```python
from build123d import *

# Parameters (mm, degrees)
BOSS_EXTRUDE3_DEPTH = 30
BOSS_EXTRUDE5_DEPTH = 13
SKETCH6_R           = 6.5
CUT_EXTRUDE1_DEPTH  = 13
SKETCH7_R           = 7.5
CUT_EXTRUDE2_DEPTH  = 13


with BuildPart() as part:
    # Sketch2 → Boss-Extrude3 (new body)
    with BuildSketch(Plane(origin=(0, 0, 0), x_dir=(0, 0, -1), z_dir=(1, 0, 0))):
        Polygon((0, 0), (0, 37), (-13, 37), (-13, 13), (-43, 13), (-43, 0), align=None)
    extrude(amount=BOSS_EXTRUDE3_DEPTH)

    # Sketch4 → Boss-Extrude5 (add)
    with BuildSketch(Plane(origin=(0, 13, 0), x_dir=(1, 0, 0), z_dir=(0, 1, 0))):
        with BuildLine():
            Line((0, -13), (0, -43))
            Line((0, -43), (-5, -43))
            ThreePointArc((-5, -43), (-20, -28), (-5, -13))
            Line((-5, -13), (0, -13))
        make_face()
    extrude(amount=-BOSS_EXTRUDE5_DEPTH)

    # Sketch6 → Cut-Extrude1 (cut)
    with BuildSketch(Plane(origin=(0, 13, 0), x_dir=(1, 0, 0), z_dir=(0, 1, 0))):
        with Locations(Location((-5, -28, 0), (0, 0, 270))):
            Circle(SKETCH6_R)
    extrude(amount=-CUT_EXTRUDE1_DEPTH, mode=Mode.SUBTRACT)

    # Sketch7 → Cut-Extrude2 (cut)
    with BuildSketch(Plane.XY.offset(13)):
        with Locations((15, 25)):
            Circle(SKETCH7_R)
    extrude(amount=-CUT_EXTRUDE2_DEPTH, mode=Mode.SUBTRACT)


solid = part.part
```
Geometry check sheet. Reference: the model listing, model coordinates, mm. A direction names the side the tool comes from. Coordinates: 2 decimals unless noted, no trailing zeros. Order: outer loops, then holes, each group sorted by start corner. A loop starts at its lowest first (then second) coordinate and runs counter-clockwise, first axis right, second up.
Q1. Thickness scan on probe 1 along Y at (x, z) = (15, 4); probe 2 along X at (y, z) = (4.25, 28); probe 3 along Y at (x, z) = (27.5, 39). Record the ranges inside material, lowest first.
Reply:
probe 1: y = 0 to 17.5, 32.5 to 37
probe 2: x = -20 to -11.5, 1.5 to 30
probe 3: y = 0 to 13
Q2. Sectioned sample at B-B on z = 28. Record the cut outline in (x, y).
Reply:
outline: (-20, 0) - (-11.5, 0) - (-11.5, 13) - (-20, 13) - close; (1.5, 0) - (30, 0) - (30, 13) - (1.5, 13) - close
Q3. Sectioned sample at D-D on y = 7.5. Record the cut outline in (x, z).
Reply:
outline: (-5, 13) - (0, 13) - (0, 0) - (30, 0) - (30, 43) - (-5, 43) arc R15 ccw to start; hole circle Ø13 at (-5, 28)
Q4. Sectioned sample at C-C on x = 15. Record the cut outline in (y, z).
Reply:
outline: (0, 0) - (17.5, 0) - (17.5, 13) - (13, 13) - (13, 43) - (0, 43) - close; (32.5, 0) - (37, 0) - (37, 13) - (32.5, 13) - close
Q5. Draft check along X on faces 4 (the face through (30, 11, 17)), 5 (the face through (11, 0, 21)), 6 (the face through (14.024, 32.436, 6.591)), 7 (the face through (-20, 7, 28)). Enter one of: released by +X, released by -X, zero draft, split by the parting line, or undercut.
Reply:
face 4: released by +X
face 5: zero draft
face 6: undercut
face 7: released by -X
Q6. Depth check by flat-ended pin: pin 1 Ø4 at (x, y) = (6, 3.5) entering from -Z; pin 2 Ø10.5 at (y, z) = (11, 4) entering from -X. Enter the tip coordinate at first touch or a pass-through.
Reply:
pin 1: stops at z = 0
pin 2: stops at x = 0
Q7. Tool access check on faces 1 (the face through (-4.714, 6.591, 21.506)), 2 (the face through (-3, 7, 13)), 3 (the face through (5, 13, 28)). Record the directions out of +Z, -Z, +X, -X, +Y, -Y that give a thin tool (end or side, any length) a straight path to the whole face; none if there is none.
Reply:
face 1: +Y, -Y
face 2: -Z, -X, +Y, -Y
face 3: +Z, +X, -X, +Y
Q8. Sectioned sample at A-A on y = 19. Record the cut outline in (x, z), and give its area (3 significant figures).
Reply:
outline: (0, 0) - (10.5, 0) - (10.5, 13) - (0, 13) - close; (19.5, 0) - (30, 0) - (30, 13) - (19.5, 13) - close
area: 273 mm2
